```python
from build123d import *

# Parameters (mm, degrees)
SKETCH_3_R        = 16
EXTRUDE_417_DEPTH = 60
SKETCH_4_R        = 15
EXTRUDE_1_DEPTH   = 60
SKETCH_9_R        = 18.5
EXTRUDE_2_DEPTH   = 10
EXTRUDE_5_DEPTH   = 10
EXTRUDE_START     = 25
SKETCH_13_R       = 16
EXTRUDE_6_DEPTH   = 25
EXTRUDE_7_DEPTH   = 10


with BuildPart() as part:
    # Эскиз3 → Extrude 417 (new body)
    with BuildSketch(Plane.XY):
        Circle(SKETCH_3_R)
    extrude(amount=EXTRUDE_417_DEPTH)

    # Эскиз4 → Бобышка-Вытянуть1 (add)
    with BuildSketch(Plane(origin=(0, 0, 0), x_dir=(1, 0, 0), z_dir=(0, -0.707106781186544, 0.7071067811865511))):
        with Locations(Location((0, 0, 0), (0, 0, 158.211329465))):
            Circle(SKETCH_4_R)
    extrude(amount=EXTRUDE_1_DEPTH)

    # Эскиз9 → Бобышка-Вытянуть2 (add)
    with BuildSketch(Plane(origin=(0, -42.426406871, 42.426406871), x_dir=(1, 0, 0), z_dir=(0, -0.7071067811865441, 0.7071067811865509))):
        with Locations(Location((0, 0, 0), (0, 0, 270))):
            Circle(SKETCH_9_R)
    extrude(amount=EXTRUDE_2_DEPTH)

    # Эскиз12 → Бобышка-Вытянуть5 (add)
    with BuildSketch(Plane.XY.offset(60)):
        Polygon((0, 20), (-17.320508076, 10), (-17.320508076, -10), (0, -20), (17.320508076, -10), (17.320508076, 10), align=None)
    extrude(amount=EXTRUDE_5_DEPTH)

    # Эскиз13 → Бобышка-Вытянуть6 (add)
    with BuildSketch(Plane(origin=(0, 0, 0), x_dir=(-1, 0, 0), z_dir=(0, 0, -1)).offset(EXTRUDE_START)):
        Circle(SKETCH_13_R)
    extrude(amount=-EXTRUDE_6_DEPTH)

    # Эскиз14 → Бобышка-Вытянуть7 (add)
    with BuildSketch(Plane(origin=(0, 0, -25), x_dir=(-1, 0, 0), z_dir=(0, 0, -1))):
        Polygon((0, -20), (17.320508076, -10), (17.320508076, 10), (0, 20), (-17.320508076, 10), (-17.320508076, -10), align=None)
    extrude(amount=EXTRUDE_7_DEPTH)


solid = part.part
```
CAD build for the part. Positions are in the model's coordinates, mm. A direction names the side the tool comes from. Give positions to 0.01 mm unless a question says otherwise; leave off trailing zeros. Order: outer loops, then holes, each group sorted by start corner. A loop starts at its lowest first (then second) coordinate and runs counter-clockwise, first axis right, second up. Notation, with made-up numbers: M -18.5,-17.75 L 31.5,-17.75 A26 cw 31.5,21.25 Z; hole C 32,-23 d5. An arc over 180 degrees is marked long. Put each result on its own line as item: value. Start each with the question number.
(1) Saw through at A-A, the plane y = 0. Write the cut outline in (x, z), then the cut area to 3 significant figures.
(2) Flat gauge pins, fed straight in: pin 1 Ø11 at (y, z) = (-3, 62.5) entering from +X; pin 2 Ø8 at (x, z) = (11, 19) entering from -Y; pin 3 Ø3 at (y, z) = (3.5, -29.5) entering from -X. Where does each tip first touch, or does it go through?
(3) Which spindle directions (+Z, -Z, +X, -X, +Y, -Y) get a long thin tool onto all of the face, cutting with end or side? Do faces 1 (the flat face through (8.78, -14.93, -29.93)), 2 (the flat face through (-8.54, -15.07, -29.93)), 3 (the flat face through (-6, -15, 60)), 4 (the flat face through (0, 0, -35)). Say none if no direction does.
(4) Saw through at C-C, the plane x = 10. Write the cut outline in (y, z).
(5) Drill centre lines: line 1 along Z through (x, y) = (-16, -9); line 2 along Y through (x, z) = (9.5, 53); line 3 along Y through (x, z) = (-8, 55.5). Where is each one in solid material? Low to high.
(6) Mould opens along Z. For faces 5 (the flat face through (8.78, 14.93, 64.93)), 6 (the flat face through (6, -15, -25)), 7 (the flat face through (0, 0, 70)) say: +Z half, -Z half, draft (parallel to the pull), parting line (faces both ways), or undercut.
(7) Saw through at B-B, the plane x = -5.5. Write the cut outline in (y, z).
Check result:
1. outline: M -17.32,-35 L 17.32,-35 L 17.32,-25 L 16,-25 L 16,60 L 17.32,60 L 17.32,70 L -17.32,70 L -17.32,60 L -16,60 L -16,-25 L -17.32,-25 Z
1. area: 3,410 mm2
2. pin 1: stops at x = 17.32
2. pin 2: stops at y = -39.62
2. pin 3: stops at x = -17.32
3. face 1: -Z, +X, -Y
3. face 2: -Z, -X, -Y
3. face 3: none
3. face 4: -Z, +X, -X, +Y, -Y
4. outline: M -60.5,38.49 L -53.43,31.42 L -50.33,34.52 L -12.49,-3.32 L -12.49,-25 L -14.23,-25 L -14.23,-35 L 14.23,-35 L 14.23,-25 L 12.49,-25 L 12.49,60 L 14.23,60 L 14.23,70 L -14.23,70 L -14.23,60 L -12.49,60 L -12.49,28.3 L -34.52,50.33 L -31.42,53.43 L -38.49,60.5 Z
5. line 1: z = -35 to -25, 60 to 70
5. line 2: y = -45.99 to -31.85, -12.87 to 12.87
5. line 3: y = -43.49 to -31.91, -13.86 to 13.86
6. face 5: draft
6. face 6: undercut
6. face 7: +Z half
7. outline: M -61.99,37.01 L -54.92,29.94 L -52.29,32.56 L -15.02,-4.71 L -15.02,-25 L -16.82,-25 L -16.82,-35 L 16.82,-35 L 16.82,-25 L 15.02,-25 L 15.02,60 L 16.82,60 L 16.82,70 L -16.82,70 L -16.82,60 L -15.02,60 L -15.02,34.76 L -32.56,52.29 L -29.94,54.92 L -37.01,61.99 Z
